Could you check a few things on this model? Use its own coordinates, in mm. A direction names the side the tool comes from. Round coordinates to 2 decimals unless told otherwise and drop trailing zeros. Write each loop counter-clockwise with the first axis right and the second up, starting at its lowest first coordinate (ties: lowest second). Pieces come first, ordered by that corner, then holes. Notation, with made-up numbers: (31.5, 3.25) -> (55.5, 3.25) arc R7 cw to (55.5, 16.25) -> close; hole circle Ø4 at (-14, 44). An arc over 180 degrees is marked (long way). One line per question, with ' | ' between items. Start each with the question number.
1. Imagine slicing it at B-B, the plane z = 3.5. List the corners of the cut face in (x, y) for me.
2. For faces 1 (the flat face through (2.5, 8, 3)), 2 (the flat face through (0, 0, 3)), 3 (the flat face through (2.8, -8, 3)), 4 (the flat face through (-2.8, 8, 3)), which set-ups out of +Z, -Z, +X, -X, +Y, -Y let a thin tool reach every point of the face, with its end or its side?
3. For pin 1 Ø0.8 at (y, z) = (-6.5, 3) entering from +X; pin 2 Ø1 at (x, y) = (0, -2) entering from -Z; pin 3 Ø2.5 at (x, y) = (0.5, 9) entering from +Z; pin 4 Ø1 at (x, y) = (0.5, 4) entering from -Z, each with a flat end and sliding along its axis, tell me the tip position at first contact or that it passes through.
4. Imagine slicing it at C-C, the plane x = 0. List the corners of the cut face in (y, z) for me.
5. Imagine slicing it at A-A, the plane y = 0. List the corners of the cut face in (x, z) for me.
6. Thinking about a two-plate mould opening in X: for faces 5 (the cylindrical face through (-0.29, 2.23, 1.48)), 6 (the cylindrical face through (-2.215, -14.699, 3.01)), 7 (the cylindrical face through (2.215, 14.699, 3.01)), 8 (the flat face through (0, -8, 2.25)), which applies, released by +X, released by -X, zero draft, split by the parting line, or undercut?
7. Imagine slicing it at D-D, the plane z = 0.45. List the corners of the cut face in (x, y) for me, and give its area (3 significant figures).
8. If I drill on line 1 along Y through (x, z) = (0, 0.7); line 2 along X through (y, z) = (-9.5, 3.35); line 3 along Z through (x, y) = (2.5, -9), over which ranges is the centre line in solid material (lowest first)? Write a range as [from, to].
from build123d import *

# Parameters (mm, degrees)
CYLINDER008_R             = 2.25
CYLINDER008_DEPTH         = 3
BOX003_W                  = 5.3
BOX003_H                  = 13.5
BOX003_DEPTH              = 1.5
FILLET002_R               = 1
FILLET002_PLACEMENT_ANGLE = 180
BOX002_W                  = 5.3
BOX002_H                  = 13.5
BOX002_DEPTH              = 1.5
FILLET001_R               = 1
CYLINDER007_R             = 3.5
CYLINDER007_DEPTH         = 3.85


with BuildPart() as cylinder008:
    # Cylinder008 → Cylinder008 (new body)
    with BuildSketch(Plane.XY):
        Circle(CYLINDER008_R)
    extrude(amount=CYLINDER008_DEPTH)


with BuildPart() as fillet002:
    # Box003 → Box003 (new body)
    with BuildSketch(Plane(origin=(-2.5, -15, 2.25), x_dir=(1, 0, 0), z_dir=(0, 0, 1))):
        with Locations((2.65, 6.75)):
            Rectangle(BOX003_W, BOX003_H)
    extrude(amount=BOX003_DEPTH)

    # Fillet002
    fillet002_edges = [fillet002.edges().sort_by_distance(p)[0] for p in [
        (-2.5, -15, 3),
        (2.8, -15, 3),
    ]]
    fillet(fillet002_edges, radius=FILLET002_R)


with BuildPart() as fillet002_1:
    # Fillet002 placement: moved
    add(fillet002.part.rotate(Axis((0, 0, 0), (0, 0, 1)), FILLET002_PLACEMENT_ANGLE))


with BuildPart() as fillet001:
    # Box002 → Box002 (new body)
    with BuildSketch(Plane(origin=(-2.5, -15, 2.25), x_dir=(1, 0, 0), z_dir=(0, 0, 1))):
        with Locations((2.65, 6.75)):
            Rectangle(BOX002_W, BOX002_H)
    extrude(amount=BOX002_DEPTH)

    # Fillet001
    fillet001_edges = [fillet001.edges().sort_by_distance(p)[0] for p in [
        (-2.5, -15, 3),
        (2.8, -15, 3),
    ]]
    fillet(fillet001_edges, radius=FILLET001_R)


with BuildPart() as servoarmdouble:
    # Cylinder007 → Cylinder007 (new body)
    with BuildSketch(Plane.XY):
        Circle(CYLINDER007_R)
    extrude(amount=CYLINDER007_DEPTH)

    # Fusion004: union Fillet002, Fillet001
    add(fillet002_1.part)
    add(fillet001.part)

    # Cut002: cut Cylinder008
    add(cylinder008.part, mode=Mode.SUBTRACT)


solid = servoarmdouble.part
Geometry results:
1) outline: (-2.8, 2.1) arc R3.5 ccw to (-2.5, -2.45) -> (-2.5, -14) arc R1 ccw to (-1.5, -15) -> (1.8, -15) arc R1 ccw to (2.8, -14) -> (2.8, -2.1) arc R3.5 ccw to (2.5, 2.45) -> (2.5, 14) arc R1 ccw to (1.5, 15) -> (-1.8, 15) arc R1 ccw to (-2.8, 14) -> close
2) face 1: +Z, -Z, +X, +Y | face 2: -Z | face 3: +Z, -Z, +X, -Y | face 4: +Z, -Z, -X, +Y
3) pin 1: stops at x = 2.8 | pin 2: stops at z = 0 | pin 3: stops at z = 3.75 | pin 4: stops at z = 2.25
4) outline: (-15, 2.25) -> (-3.5, 2.25) -> (-3.5, 0) -> (-2.25, 0) -> (-2.25, 3) -> (2.25, 3) -> (2.25, 0) -> (3.5, 0) -> (3.5, 2.25) -> (15, 2.25) -> (15, 3.75) -> (3.5, 3.75) -> (3.5, 3.85) -> (-3.5, 3.85) -> (-3.5, 3.75) -> (-15, 3.75) -> close
5) outline: (-3.5, 0) -> (-2.25, 0) -> (-2.25, 3) -> (2.25, 3) -> (2.25, 0) -> (3.5, 0) -> (3.5, 3.85) -> (-3.5, 3.85) -> close
6) face 5: undercut | face 6: released by -X | face 7: released by +X | face 8: zero draft
7) outline: circle Ø7 at (0, 0); hole circle Ø4.5 at (0, 0) | area: 22.6 mm2
8) line 1: y = [-3.5, -2.25], [2.25, 3.5] | line 2: x = [-2.5, 2.8] | line 3: z = [2.25, 3.75]
